Geometry: final body of the model. Coordinates: model frame, mm. Face numbers are marked on the shaded views. Give positions to 0.01 mm unless a question says otherwise; leave off trailing zeros. Loops run counter-clockwise (first coordinate to the right, second up) from the corner with the lowest first, then second, coordinate; pieces in that order, holes last.
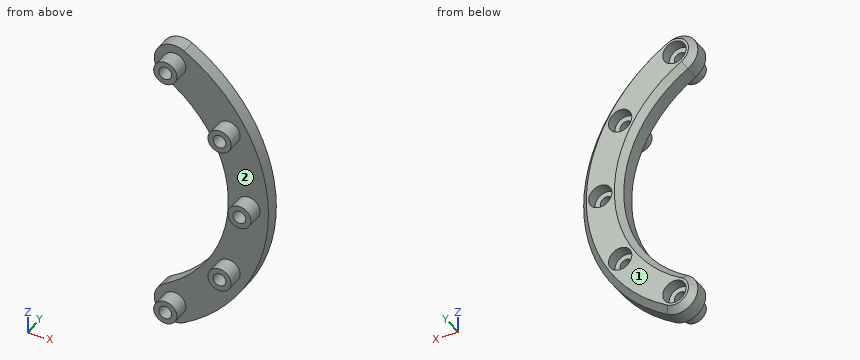
from build123d import *

# Parameters (mm, degrees)
EXTRUDE_1_DEPTH     = 5
SKETCH_3_R          = 2.9
EXTRUDE_3_DEPTH     = 4
SKETCH_4_R          = 1.6
CUT_EXTRUDE_1_DEPTH = 10
SKETCH_5_R          = 2.9
CUT_EXTRUDE_2_DEPTH = 2.8
CHAMFER_1_SIZE      = 1.5


with BuildPart() as part:
    # 草图1 → 凸台-拉伸1 (new body)
    with BuildSketch(Plane(origin=(0, 0, 0), x_dir=(1, 0, 0), z_dir=(0, 1, 0))):
        with BuildLine():
            ThreePointArc((21, -36.373066959), (14.169872981, -34.54293994), (16, -27.712812921))
            ThreePointArc((16, -27.712812921), (32, 0), (16, 27.712812921))
            ThreePointArc((16, 27.712812921), (14.169872981, 34.54293994), (21, 36.373066959))
            ThreePointArc((21, 36.373066959), (42, 0), (21, -36.373066959))
        make_face()
    extrude(amount=EXTRUDE_1_DEPTH)

    # 草图3 → 凸台-拉伸3 (add)
    with BuildSketch(Plane.XZ):
        with Locations((18.5, 32.04293994)):
            Circle(SKETCH_3_R)
        with Locations((32.04293994, 18.5)):
            Circle(SKETCH_3_R)
        with Locations((37, 0)):
            Circle(SKETCH_3_R)
        with Locations((32.04293994, -18.5)):
            Circle(SKETCH_3_R)
        with Locations((18.5, -32.04293994)):
            Circle(SKETCH_3_R)
    extrude(amount=EXTRUDE_3_DEPTH)

    # 草图4 → 切除-拉伸1 (cut, through all)
    with BuildSketch(Plane(origin=(0, 5, 0), x_dir=(1, 0, 0), z_dir=(0, 1, 0))):
        with Locations((18.5, 32.04293994)):
            Circle(SKETCH_4_R)
        with Locations((32.04293994, 18.5)):
            Circle(SKETCH_4_R)
        with Locations((37, 0)):
            Circle(SKETCH_4_R)
        with Locations((32.04293994, -18.5)):
            Circle(SKETCH_4_R)
        with Locations((18.5, -32.04293994)):
            Circle(SKETCH_4_R)
    extrude(amount=-CUT_EXTRUDE_1_DEPTH, mode=Mode.SUBTRACT)

    # 草图5 → 切除-拉伸2 (cut)
    with BuildSketch(Plane(origin=(0, 5, 0), x_dir=(1, 0, 0), z_dir=(0, 1, 0))):
        with Locations((18.5, 32.04293994)):
            Circle(SKETCH_5_R)
        with Locations((32.04293994, 18.5)):
            Circle(SKETCH_5_R)
        with Locations((37, 0)):
            Circle(SKETCH_5_R)
        with Locations((32.04293994, -18.5)):
            Circle(SKETCH_5_R)
        with Locations((18.5, -32.04293994)):
            Circle(SKETCH_5_R)
    extrude(amount=-CUT_EXTRUDE_2_DEPTH, mode=Mode.SUBTRACT)

    # 倒角1
    chamfer_1_edges = [part.edges().sort_by_distance(p)[0] for p in [
        (42, 5, 0),
        (14.169872981, 5, -34.54293994),
        (32, 5, 0),
        (14.169872981, 5, 34.54293994),
    ]]
    chamfer(chamfer_1_edges, length=CHAMFER_1_SIZE)


solid = part.part
Item 1: Draft query along Z for the marked faces 1 and 2. Return one class per face: +Z half, -Z half, draft (parallel to the pull), parting line (faces both ways), or undercut.
Values follow:
face 1: draft
face 2: undercut
Item 2: Section query B-B on y = 4.25. Return loops of the section in (x, z) (3 decimals), plus the area to 3 significant figures.
Values follow:
outline: (16.375, -28.362) arc R4.25 ccw to (20.625, -35.724) arc R41.25 ccw to (20.625, 35.724) arc R4.25 ccw to (16.375, 28.362) arc R32.75 cw to start; hole circle Ø5.8 at (18.5, -32.043); hole circle Ø5.8 at (18.5, 32.043); hole circle Ø5.8 at (32.043, -18.5); hole circle Ø5.8 at (32.043, 18.5); hole circle Ø5.8 at (37, 0)
area: 583 mm2
Item 3: Pin query (flat end, axial travel): pin 1 (3 mm diameter, centred on x = 32.04, z = -18.5, fed in from +Y); pin 2 (3 mm diameter, centred on x = 36.5, z = 1, fed in from +Y); pin 3 (1.5 mm diameter, centred on x = 33.5, z = -3.5, fed in from -Y). Return the tip coordinate at first contact, or that it passes through.
Values follow:
pin 1: passes through
pin 2: stops at y = 2.2
pin 3: stops at y = 0
Item 4: Section query A-A on y = -2.75. Give the number of separate pieces and of enclosed holes in the cut face, plus the area to 3 significant figures.
Values follow:
separate pieces: 5
enclosed holes: 5
area: 91.9 mm2
Item 5: Ray query, probe 1 along Z at (x, y) = (18.5, -2); probe 2 along Z at (x, y) = (32, -2.25); probe 3 along X at (y, z) = (-3, -31). Return the intervals inside material, ascending.
Values follow:
probe 1: z = -34.94 to -33.64, -30.44 to -29.14, 29.14 to 30.44, 33.64 to 34.94
probe 2: z = -21.4 to -20.1, -16.9 to -15.6, 15.6 to 16.9, 20.1 to 21.4
probe 3: x = 15.79 to 17.29, 19.71 to 21.21
